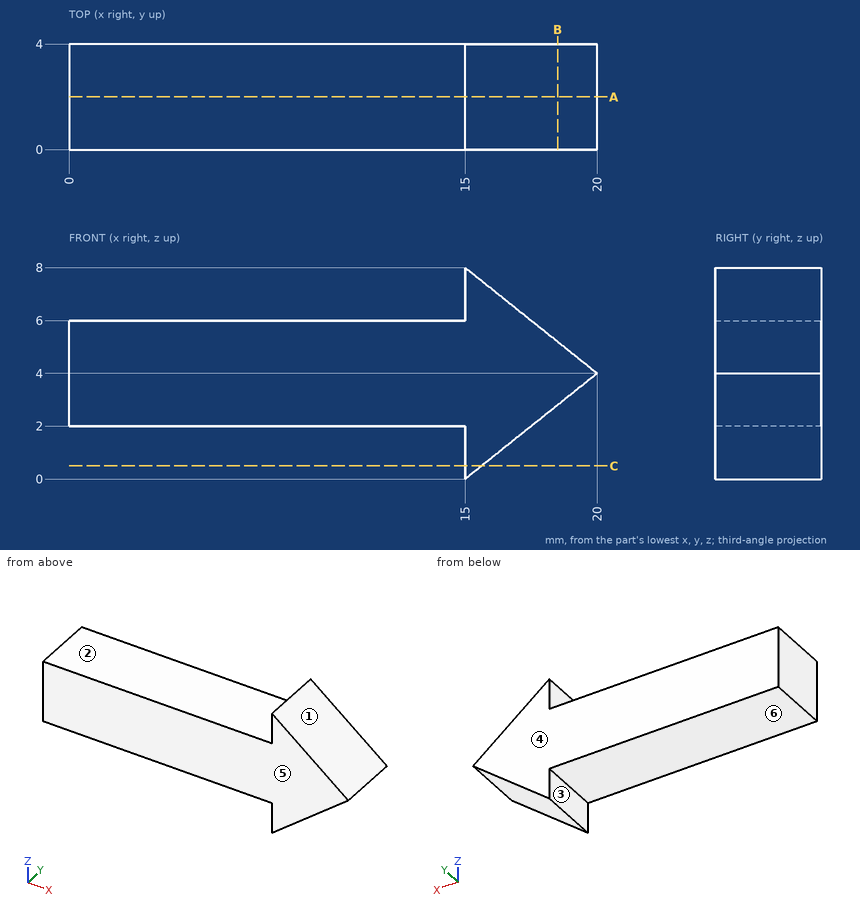
Geometry check sheet. Reference: drawing and pictorial views, mm from the part's lowest x, y, z. A direction names the side the tool comes from. Round coordinates to 2 decimals unless told otherwise and drop trailing zeros. Loops run counter-clockwise (first coordinate to the right, second up) from the corner with the lowest first, then second, coordinate; pieces in that order, holes last. Notation, with made-up numbers: (57, 63) - (110, 63) arc R12 ccw to (110, 84) - close; hole circle Ø2 at (65.5, 47.25). An arc over 180 degrees is marked (long way). One line per question, with ' | ' between items. Start each with the question number.
1. Cross-section at C-C on z = 0.5. Record the cut outline in (x, y) (3 decimals).
2. Cross-section at A-A on y = 2. Record the cut outline in (x, z).
3. Draft check along Y on the marked faces 4, 5 and 6. Enter one of: released by +Y, released by -Y, zero draft, split by the parting line, or undercut.
4. Scan lines: line 1 (Z direction, x = 5.75, y = 2.35); line 2 (Z direction, x = 17, y = 0.8); line 3 (X direction, y = 1.95, z = 5.5) (3 decimals). Record each from-to range of solid material in increasing order. Write a range as [from, to].
5. Depth check by flat-ended pin: pin 1 (4 mm diameter, centred on x = 2.5, z = 3.5, fed in from -Y); pin 2 (2 mm diameter, centred on x = 11, y = 1.5, fed in from -Z); pin 3 (2 mm diameter, centred on y = 1, z = 0.5, fed in from -X); pin 4 (1.2 mm diameter, centred on x = 10, y = 1.5, fed in from +Z). Enter the tip coordinate at first touch or a pass-through.
6. Tool access check on the marked faces 1, 2 and 3. Record the directions out of +Z, -Z, +X, -X, +Y, -Y that give a thin tool (end or side, any length) a straight path to the whole face; none if there is none.
7. Cross-section at B-B on x = 18.5. Record the cut outline in (y, z), then the cut area to 3 significant figures.
Taken from the geometry:
1) outline: (15, 0) - (15.625, 0) - (15.625, 4) - (15, 4) - close
2) outline: (0, 2) - (15, 2) - (15, 0) - (20, 4) - (15, 8) - (15, 6) - (0, 6) - close
3) face 4: released by +Y | face 5: released by -Y | face 6: zero draft
4) line 1: [2, 6] | line 2: [1.6, 6.4] | line 3: [0, 18.125]
5) pin 1: y = 0 | pin 2: z = 2 | pin 3: x = 15 | pin 4: z = 6
6) face 1: +Z, +X, +Y, -Y | face 2: +Z, -X, +Y, -Y | face 3: -Z, -X, +Y, -Y
7) outline: (0, 2.8) - (4, 2.8) - (4, 5.2) - (0, 5.2) - close | area: 9.60 mm²
